Verification items for this drawing (mm, ordinates from the low corner). Coordinates: 2 decimals unless noted, no trailing zeros. Order: outer loops, then holes, each group sorted by start corner. A loop starts at its lowest first (then second) coordinate and runs counter-clockwise, first axis right, second up. Notation, with made-up numbers: M 55.25,21.5 L 77.25,21.5 A31 ccw 77.25,49.5 Z; hole C 78.5,63 d10. An arc over 180 degrees is marked long. One line per item, written item: value. Start each with the question number.
1) Sectioned sample at D-D, the plane z = 95.5. Enter the section's corners in (x, y), then the cut area to 3 significant figures.
2) Sectioned sample at C-C, the plane z = 63. Enter the section's corners in (x, y), then the cut area to 3 significant figures.
3) Go/stop test with flat-tipped pins: P1, Ø3, axis at x = 37.5, z = 29, coming from the +Y side; P2, Ø8, axis at y = 41, z = 33.5, coming from the +X side; P3, Ø3, axis at x = 42, z = 58.5, coming from the +Y side. Record where each tip stops, or that it passes through.
4) Thickness scan on L1, parallel to X at y = 39, z = 39.5; L2, parallel to Y at x = 5, z = 35; L3, parallel to X at y = 14.5, z = 15. Record the ranges inside material, lowest first. Write a range as from..to.
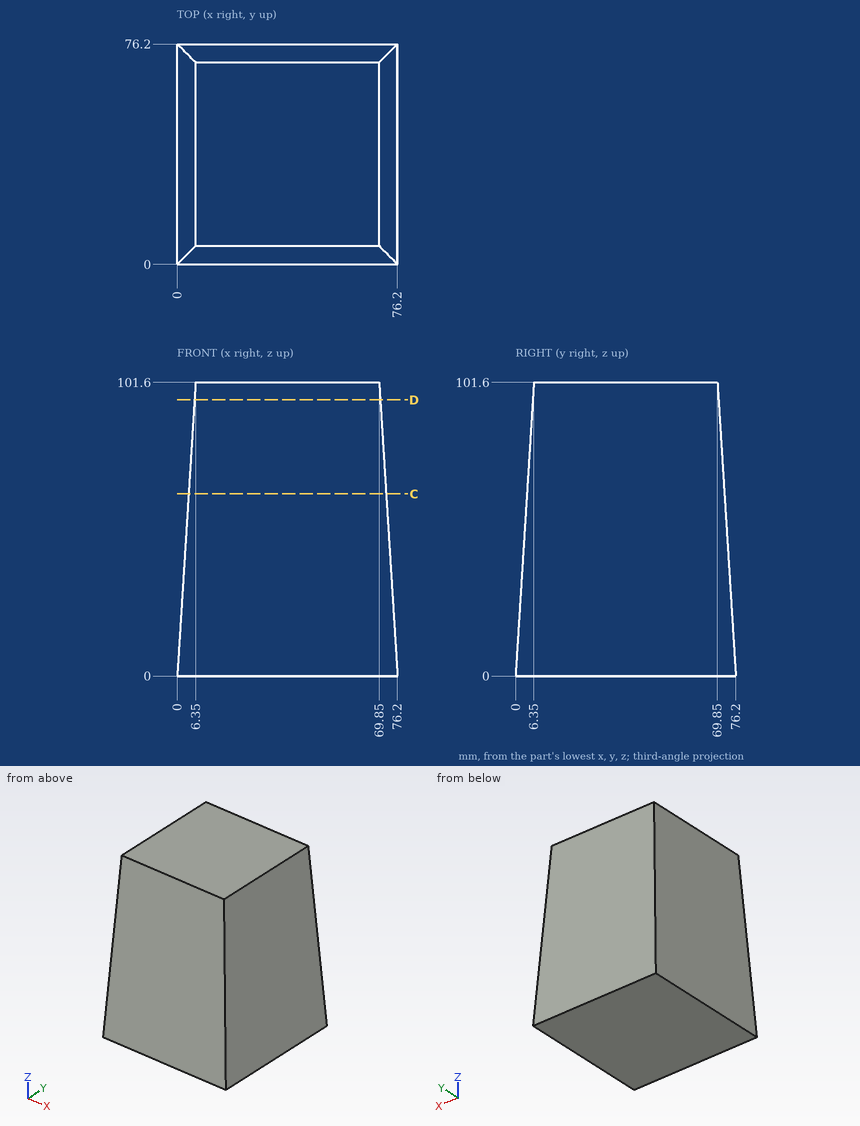
Final values:
1. outline: M 5.97,5.97 L 70.23,5.97 L 70.23,70.23 L 5.97,70.23 Z
1. area: 4,130 mm^2
2. outline: M 3.94,3.94 L 72.26,3.94 L 72.26,72.26 L 3.94,72.26 Z
2. area: 4,670 mm^2
3. P1: stops at y = 74.48
3. P2: stops at x = 74.36
3. P3: stops at y = 72.64
4. L1: x = 2.47..73.73
4. L2: y = 2.19..74.01
4. L3: x = 0.94..75.26
